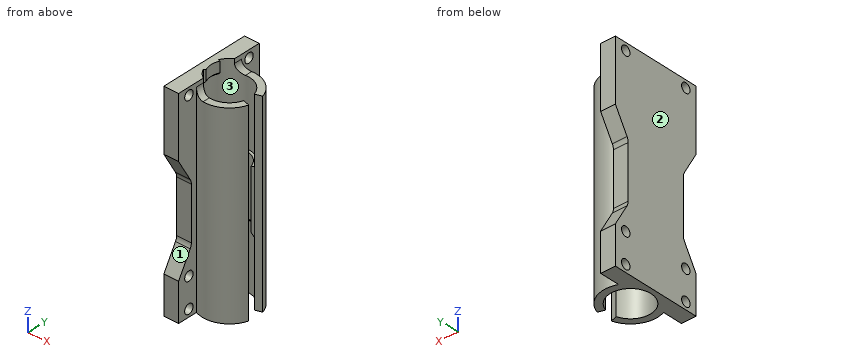
```python
from build123d import *

# Parameters (mm, degrees)
BOSS_EXTRUDE1_DEPTH      = 98
SKETCH2_R                = 2.25
CUT_EXTRUDE1_DEPTH       = 25.44661253
SKETCH4_W                = 19.691623847
SKETCH4_H                = 43
CUT_EXTRUDE2_DEPTH       = 6
FILLET1_R                = 4
CUT_EXTRUDE3_DEPTH       = 62.0000001
CUT_EXTRUDE4_DEPTH       = 25.44661263
REVOLVE2_ANGLE           = 25
REVOLVE2_OTHER_WAY_ANGLE = 25


with BuildPart() as part:
    # Sketch1 → Boss-Extrude1 (new body)
    with BuildSketch(Plane.XY):
        with BuildLine():
            Line((-5, -12), (-5, -21.5))
            Line((-5, -21.5), (-12, -21.5))
            Line((-12, -21.5), (-12, 21.5))
            Line((-12, 21.5), (-5, 21.5))
            Line((-5, 21.5), (-5, 12))
            ThreePointArc((-5, 12), (5.555898195, 11.752956872), (12.44661253, 3.75257732))
            Line((12.44661253, 3.75257732), (9.287087811, 2.8))
            ThreePointArc((9.287087811, 2.8), (-9.7, 0), (9.287087811, -2.8))
            Line((9.287087811, -2.8), (12.44661253, -3.75257732))
            ThreePointArc((12.44661253, -3.75257732), (5.555898195, -11.752956872), (-5, -12))
        make_face()
    extrude(amount=BOSS_EXTRUDE1_DEPTH)

    # Sketch2 → Cut-Extrude1 (cut, through all)
    with BuildSketch(Plane.ZY.offset(12)):
        with Locations((3.5, 16)):
            Circle(SKETCH2_R)
        with Locations((94.5, -16)):
            Circle(SKETCH2_R)
        with Locations((94.5, 16)):
            Circle(SKETCH2_R)
        with Locations((3.5, -16)):
            Circle(SKETCH2_R)
        with Locations((17.5, 16)):
            Circle(SKETCH2_R)
        with Locations((17.5, -16)):
            Circle(SKETCH2_R)
    extrude(amount=-CUT_EXTRUDE1_DEPTH, mode=Mode.SUBTRACT)

    # Sketch3 → Revolve1 (revolve)
    with BuildSketch(Plane.ZY, mode=Mode.PRIVATE) as revolve1_sk:
        Polygon((31, 9.7), (32.713777608, 8.5), (61, 8.5), (61, 9.7), align=None)
    revolve(revolve1_sk.sketch.rotate(Axis((0, 0, 0), (0, 0, 1)), 90), axis=Axis((0, 0, 0), (0, 0, 1)))  # turned: the seam where the file's is

    # Sketch4 → Cut-Extrude2 (cut)
    with BuildSketch(Plane.XY.offset(98)):
        with Locations((4.845811924, 0)):
            Rectangle(SKETCH4_W, SKETCH4_H)
    extrude(amount=-CUT_EXTRUDE2_DEPTH, mode=Mode.SUBTRACT)

    # Fillet1
    fillet1_edges = [part.edges().sort_by_distance(p)[0] for p in [
        (-5, 10.15601973, 92),
        (-5, -10.15601973, 92),
    ]]
    fillet(fillet1_edges, radius=FILLET1_R)

    # Sketch5 → Cut-Extrude3 (cut, through all)
    with BuildSketch(Plane.XY.offset(61)):
        with BuildLine():
            Line((8.138169731, 2.453608247), (9.287087811, 2.8))
            ThreePointArc((9.287087811, 2.8), (9.7, 0), (9.287087811, -2.8))
            Line((9.287087811, -2.8), (8.138169731, -2.453608247))
            ThreePointArc((8.138169731, -2.453608247), (8.5, 0), (8.138169731, 2.453608247))
        make_face()
    extrude(amount=-CUT_EXTRUDE3_DEPTH, mode=Mode.SUBTRACT)

    # Sketch6 → Cut-Extrude4 (cut, through all)
    with BuildSketch(Plane.ZY.offset(12)):
        with BuildLine():
            Line((28.75, 15.302885683), (18.016283143, 21.5))
            Line((18.016283143, 21.5), (68.983716857, 21.5))
            Line((68.983716857, 21.5), (58.25, 15.302885683))
            ThreePointArc((58.25, 15.302885683), (57.164685703, 14.853333782), (56, 14.7))
            Line((56, 14.7), (31, 14.7))
            ThreePointArc((31, 14.7), (29.835314297, 14.853333782), (28.75, 15.302885683))
        make_face()
    cut_extrude4 = extrude(amount=-CUT_EXTRUDE4_DEPTH, mode=Mode.SUBTRACT)

    # Mirror1: Cut-Extrude4 across plane
    add(cut_extrude4.mirror(Plane.ZX), mode=Mode.SUBTRACT)

    # Sketch7 → Revolve2 (revolve)
    with BuildSketch(Plane(origin=(0, 0, 0), x_dir=(1, 0, 0), z_dir=(0, 1, 0))):
        Polygon((-9.7, -92), (-9.7, -98), (-8.7, -98), (-8.7, -93), align=None)
    revolve(axis=Axis((0, 0, 97.129634248), (0, 0, -1)), revolution_arc=REVOLVE2_ANGLE)

    # Sketch7 → Revolve2 other way (revolve)
    with BuildSketch(Plane(origin=(0, 0, 0), x_dir=(1, 0, 0), z_dir=(0, 1, 0))):
        Polygon((-9.7, -92), (-9.7, -98), (-8.7, -98), (-8.7, -93), align=None)
    revolve(axis=Axis((0, 0, 97.129634248), (0, 0, 1)), revolution_arc=REVOLVE2_OTHER_WAY_ANGLE)


solid = part.part
```
For this review, take the finished solid that the model builds, in its own axes (mm). Face numbers are marked on the shaded views. Coordinates: 2 decimals unless noted, no trailing zeros. Loops run counter-clockwise (first coordinate to the right, second up) from the corner with the lowest first, then second, coordinate; pieces in that order, holes last.
1. Add section D-D, the plane z = 60. Give the boundary of the cut face in (x, y), then the cut area to 3 significant figures.
2. Add section B-B, the plane z = 80. Give the boundary of the cut face in (x, y).
3. Add section C-C, the plane z = 94.5. Give the boundary of the cut face in (x, y).
4. Insertion check: P1, Ø2, axis at x = -1, y = 9, coming from the +Z side; P2, Ø2.5, axis at y = 16, z = 17.5, coming from the -X side; P3, Ø5, axis at y = 16, z = 94.5, coming from the +X side; P4, Ø14.5, axis at y = 15.5, z = 50.5, coming from the +X side. Each pin has a flat end and moves straight along its axis. Give the tip position at first contact, or say it passes through.
5. Add section A-A, the plane y = 0. Give the boundary of the cut face in (x, z), then the cut area to 3 significant figures.
6. Mouldability with a two-part tool opening along Y and no side actions: class the marked faces 1, 2 and 3 as +Y half, -Y half, draft (parallel to the pull), parting line (faces both ways), or undercut.
7. For line 1 (Y direction, x = -9.75, z = 17.5); line 2 (Y direction, x = 0, z = 74); line 3 (Y direction, x = -3.5, z = 60), list the stretches that pass through material, from the lowest coordinate up.
Result:
1. outline: (-12, -16.31) - (-5, -16.31) - (-5, -12) arc R13 ccw to (12.45, -3.75) - (8.14, -2.45) arc R8.5 cw (long way) to (8.14, 2.45) - (12.45, 3.75) arc R13 ccw to (-5, 12) - (-5, 16.31) - (-12, 16.31) - close
1. area: 365 mm2
2. outline: (-12, -21.5) - (-5, -21.5) - (-5, -12) arc R13 ccw to (12.45, -3.75) - (9.29, -2.8) arc R9.7 cw (long way) to (9.29, 2.8) - (12.45, 3.75) arc R13 ccw to (-5, 12) - (-5, 21.5) - (-12, 21.5) - close
3. outline: (-12, -21.5) - (-5, -21.5) - (-5, -18.25) - (-12, -18.25) - close; (-12, -13.75) - (-5, -13.75) - (-5, -12) arc R13 ccw to (-4.71, -12.12) - (-4.71, -8.48) arc R9.7 cw to (-8.79, -4.1) - (-7.88, -3.68) arc R8.7 cw to (-7.88, 3.68) - (-8.79, 4.1) arc R9.7 cw to (-4.71, 8.48) - (-4.71, 12.12) arc R13 ccw to (-5, 12) - (-5, 13.75) - (-12, 13.75) - close; (-12, 18.25) - (-5, 18.25) - (-5, 21.5) - (-12, 21.5) - close
4. P1: stops at z = 92.09
4. P2: passes through
4. P3: stops at x = -5
4. P4: stops at x = 10.05
5. outline: (-12, 0) - (-9.7, 0) - (-9.7, 31) - (-8.5, 32.71) - (-8.5, 61) - (-9.7, 61) - (-9.7, 92) - (-8.7, 93) - (-8.7, 98) - (-12, 98) - close
5. area: 266 mm2
6. face 1: -Y half
6. face 2: draft
6. face 3: undercut
7. line 1: y = -21.5 to -18.25, -13.75 to 13.75, 18.25 to 21.5
7. line 2: y = -13 to -9.7, 9.7 to 13
7. line 3: y = -12.52 to -7.75, 7.75 to 12.52
